from build123d import *

# Parameters (mm, degrees)
SZKIC1_R                    = 5
DODANIE_WYCI_GNI_CIE1_DEPTH = 33
SZKIC2_R                    = 20
DODANIE_WYCI_GNI_CIE2_DEPTH = 2
SZKIC3_R                    = 44
DODANIE_WYCI_GNI_CIE3_DEPTH = 15
SZKIC5_R                    = 5
DODANIE_WYCI_GNI_CIE6_DEPTH = 20
SZKIC6_R                    = 44
DODANIE_WYCI_GNI_CIE7_DEPTH = 15
SZKIC7_R                    = 20
DODANIE_WYCI_GNI_CIE8_DEPTH = 2
SZKIC8_R                    = 5
DODANIE_WYCI_GNI_CIE9_DEPTH = 33


with BuildPart() as part:
    # Szkic1 → Dodanie-wyciągnięcie1 (new body)
    with BuildSketch(Plane.XY):
        Circle(SZKIC1_R)
    extrude(amount=-DODANIE_WYCI_GNI_CIE1_DEPTH)

    # Szkic2 → Dodanie-wyciągnięcie2 (add)
    with BuildSketch(Plane(origin=(0, 0, -33), x_dir=(-1, 0, 0), z_dir=(0, 0, -1))):
        Circle(SZKIC2_R)
    extrude(amount=DODANIE_WYCI_GNI_CIE2_DEPTH)

    # Szkic3 → Dodanie-wyciągnięcie3 (add)
    with BuildSketch(Plane(origin=(0, 0, -35), x_dir=(-1, 0, 0), z_dir=(0, 0, -1))):
        Circle(SZKIC3_R)
    extrude(amount=DODANIE_WYCI_GNI_CIE3_DEPTH)

    # Szkic5 → Dodanie-wyciągnięcie6 (add)
    with BuildSketch(Plane(origin=(0, 0, -50), x_dir=(-1, 0, 0), z_dir=(0, 0, -1))):
        with Locations((9.134986503, -17.79190888)):
            Circle(SZKIC5_R)
    extrude(amount=DODANIE_WYCI_GNI_CIE6_DEPTH)

    # Szkic6 → Dodanie-wyciągnięcie7 (add)
    with BuildSketch(Plane(origin=(0, 0, -70), x_dir=(-1, 0, 0), z_dir=(0, 0, -1))):
        Circle(SZKIC6_R)
    extrude(amount=DODANIE_WYCI_GNI_CIE7_DEPTH)

    # Szkic7 → Dodanie-wyciągnięcie8 (add)
    with BuildSketch(Plane(origin=(0, 0, -85), x_dir=(-1, 0, 0), z_dir=(0, 0, -1))):
        Circle(SZKIC7_R)
    extrude(amount=DODANIE_WYCI_GNI_CIE8_DEPTH)

    # Szkic8 → Dodanie-wyciągnięcie9 (add)
    with BuildSketch(Plane(origin=(0, 0, -87), x_dir=(-1, 0, 0), z_dir=(0, 0, -1))):
        Circle(SZKIC8_R)
    extrude(amount=DODANIE_WYCI_GNI_CIE9_DEPTH)


solid = part.part
Check sheet for the modelled part. Datum: model origin and axes. Units: mm. A direction names the side the tool comes from. Coordinates: 2 decimals unless noted, no trailing zeros. Loops run counter-clockwise (first coordinate to the right, second up) from the corner with the lowest first, then second, coordinate; pieces in that order, holes last. Notation, with made-up numbers: (-9, 63) -> (-5, 63) arc R28 cw to (-5, 84) -> close; hole circle Ø8 at (-9, -11.75). An arc over 180 degrees is marked (long way). Answer in a Markdown table with one row per item.
1. Access from +Z, -Z, +X, -X, +Y, -Y to the whole of each face (thin tool, end or side, straight path). Record for faces 1 (the face through (-9, -19, -85)), 2 (the face through (-9, -19, -35)), 3 (the face through (-11.44, -22.23, -59.86)).
Check values:
| item | result |
|---|---|
| face 1 | -Z |
| face 2 | +Z |
| face 3 | none |
2. Go/stop test with flat-tipped pins: pin 1 (6 mm diameter, centred on x = -31.5, z = -33, fed in from +Y); pin 2 (4 mm diameter, centred on x = 9, z = -70, fed in from +Y); pin 3 (10 mm diameter, centred on y = -8.5, z = -64, fed in from -X). Record where each tip stops, or that it passes through.
Check values:
| item | result |
|---|---|
| pin 1 | stops at y = 32.86 |
| pin 2 | stops at y = 43.44 |
| pin 3 | stops at x = -11.7 |
3. Sectioned sample at A-A, the plane x = 0. Record the boundary of the cut face in (y, z), then the cut area to 3 significant figures.
Check values:
| item | result |
|---|---|
| outline | (-44, -85) -> (-20, -85) -> (-20, -87) -> (-5, -87) -> (-5, -120) -> (5, -120) -> (5, -87) -> (20, -87) -> (20, -85) -> (44, -85) -> (44, -70) -> (-44, -70) -> close; (-44, -50) -> (44, -50) -> (44, -35) -> (20, -35) -> (20, -33) -> (5, -33) -> (5, 0) -> (-5, 0) -> (-5, -33) -> (-20, -33) -> (-20, -35) -> (-44, -35) -> close |
| area | 3,460 mm2 |
4. Release check for a two-part mould opening along Z. For faces 4 (the face through (1, 1, -70)), 5 (the face through (4.336, -19.524, -33.986)), 6 (the face through (-4, -4, -33)), 7 (the face through (1, 1, -50)) record: released by +Z, released by -Z, zero draft, split by the parting line, or undercut.
Check values:
| item | result |
|---|---|
| face 4 | undercut |
| face 5 | zero draft |
| face 6 | released by +Z |
| face 7 | undercut |
5. Sectioned sample at D-D, the plane z = -16. Record the boundary of the cut face in (x, y), then the cut area to 3 significant figures.
Check values:
| item | result |
|---|---|
| outline | circle Ø10 at (0, 0) |
| area | 78.5 mm2 |
6. Sectioned sample at B-B, the plane y = -33.5. Record the boundary of the cut face in (x, z).
Check values:
| item | result |
|---|---|
| outline | (-28.53, -85) -> (28.53, -85) -> (28.53, -70) -> (-28.53, -70) -> close; (-28.53, -50) -> (28.53, -50) -> (28.53, -35) -> (-28.53, -35) -> close |
7. Material ranges on line 1 along Z through (x, y) = (24, -25.5); line 2 along Z through (x, y) = (-8, 17); line 3 along Y through (x, z) = (19.5, -76.5), recorded low to high. Write a range as [from, to].
Check values:
| item | result |
|---|---|
| line 1 | z = [-85, -70], [-50, -35] |
| line 2 | z = [-87, -70], [-50, -33] |
| line 3 | y = [-39.44, 39.44] |
